from build123d import *

# Parameters (mm, degrees)
F1_DEPTH      = 76.2
F2_W          = 50.8
F2_H          = 25.4
F3_DEPTH      = 50.801
F3_DEPTH_BACK = 50.801
F5_DEPTH      = 25.4
F6_DEPTH      = 25.4
F7_W          = 25.4
F7_H          = 25.4968867362
F8_DEPTH      = 101.6
F9_R          = 12.7


with BuildPart() as f1:
    # F0 (on Top) → F1 (new body)
    with BuildSketch(Plane.XY):
        Polygon((-50.8, 101.6), (0, 0), (50.8, 101.6), align=None)
    extrude(amount=F1_DEPTH)

    # F2 (on Right) → F3 (cut, two sides)
    with BuildSketch(Plane.YZ) as f3_sk:
        with Locations((25.4, 38.1)):
            Rectangle(F2_W, F2_H)
    extrude(amount=-F3_DEPTH, mode=Mode.SUBTRACT)
    extrude(f3_sk.sketch, amount=F3_DEPTH_BACK, mode=Mode.SUBTRACT)

    # F4 (on face) → F5 (join)
    with BuildSketch(Plane(origin=(0, 0, 0), x_dir=(1, 0, 0), z_dir=(0, 0, -1))):
        with BuildLine():
            Line((63.5, -31.75), (101.6, -31.75))
            Line((101.6, -31.75), (101.6, -12.7))
            ThreePointArc((101.6, -12.7), (97.8802561211, -3.7197438789), (88.9, 0))
            Line((88.9, 0), (-88.9, 0))
            ThreePointArc((-88.9, 0), (-97.8802561211, -3.7197438789), (-101.6, -12.7))
            Line((-101.6, -12.7), (-101.6, -31.75))
            Line((-101.6, -31.75), (-63.5, -31.75))
            Line((-63.5, -31.75), (-63.5, -69.85))
            Line((-63.5, -69.85), (-101.6, -69.85))
            Line((-101.6, -69.85), (-101.6, -88.9))
            ThreePointArc((-101.6, -88.9), (-97.8802561211, -97.8802561211), (-88.9, -101.6))
            Line((-88.9, -101.6), (-50.8, -101.6))
            Line((-50.8, -101.6), (50.8, -101.6))
            Line((50.8, -101.6), (88.9, -101.6))
            ThreePointArc((88.9, -101.6), (97.8802561211, -97.8802561211), (101.6, -88.9))
            Line((101.6, -88.9), (101.6, -69.85))
            Line((101.6, -69.85), (63.5, -69.85))
            Line((63.5, -69.85), (63.5, -31.75))
        make_face()
    extrude(amount=F5_DEPTH)

    # F4 (on face) → F6 (join)
    with BuildSketch(Plane(origin=(0, 0, 0), x_dir=(1, 0, 0), z_dir=(0, 0, -1))):
        with BuildLine():
            Line((63.5, -31.75), (101.6, -31.75))
            Line((101.6, -31.75), (101.6, -12.7))
            ThreePointArc((101.6, -12.7), (97.8802561211, -3.7197438789), (88.9, 0))
            Line((88.9, 0), (-88.9, 0))
            ThreePointArc((-88.9, 0), (-97.8802561211, -3.7197438789), (-101.6, -12.7))
            Line((-101.6, -12.7), (-101.6, -31.75))
            Line((-101.6, -31.75), (-63.5, -31.75))
            Line((-63.5, -31.75), (-63.5, -69.85))
            Line((-63.5, -69.85), (-101.6, -69.85))
            Line((-101.6, -69.85), (-101.6, -88.9))
            ThreePointArc((-101.6, -88.9), (-97.8802561211, -97.8802561211), (-88.9, -101.6))
            Line((-88.9, -101.6), (-50.8, -101.6))
            Line((-50.8, -101.6), (50.8, -101.6))
            Line((50.8, -101.6), (88.9, -101.6))
            ThreePointArc((88.9, -101.6), (97.8802561211, -97.8802561211), (101.6, -88.9))
            Line((101.6, -88.9), (101.6, -69.85))
            Line((101.6, -69.85), (63.5, -69.85))
            Line((63.5, -69.85), (63.5, -31.75))
        make_face()
    extrude(amount=F6_DEPTH)

    # F7 (on face) → F8 (join)
    with BuildSketch(Plane.XZ):
        with Locations((-50.8, -38.1484433681)):
            Rectangle(F7_W, F7_H)
        with Locations((50.8, -38.1484433681)):
            Rectangle(F7_W, F7_H)
    extrude(amount=-F8_DEPTH)

    # F9
    f9_edges = [f1.edges().sort_by_distance(p)[0] for p in [
        (-38.1, 50.8, -25.4),
        (38.1, 50.8, -25.4),
    ]]
    fillet(f9_edges, radius=F9_R)


solid = f1.part
Source: CAD feature listing. Evaluate the final solid. Frame: model axes, mm. A direction names the side the tool comes from. Round coordinates to 2 decimals unless told otherwise and drop trailing zeros. Loops run counter-clockwise (first coordinate to the right, second up) from the corner with the lowest first, then second, coordinate; pieces in that order, holes last. Notation, with made-up numbers: (20, 46) - (34, 46) arc R25 cw to (34, 82) - close; hole circle Ø3 at (-22.5, 11.5). An arc over 180 degrees is marked (long way). Write item = value, one per line. Start each with the question number.
Item 1: Section query B-B on y = 47.5. Output: boundary loops of the cut face in (x, z), plus the area to 3 significant figures.
Item 2: Material intervals for line 1 (Z direction, x = -10.5, y = 25); line 2 (X direction, y = 45.5, z = -44); line 3 (Z direction, x = 7, y = 71), sorted ascending.
Item 3: Reachability of faces 4 (the face through (-26, 52, 38)), 5 (the face through (-83, 31.75, -13)), 6 (the face through (-83, 16, -25.4)), 7 (the face through (0, 31, 25.4)) from +Z, -Z, +X, -X, +Y, -Y: full face, straight path, thin tool, end or side. Return the list, or none.
Item 4: Section query C-C on y = 58.5. Output: boundary loops of the cut face in (x, z), plus the area to 3 significant figures.
Item 5: Section query A-A on x = 68. Output: boundary loops of the cut face in (y, z), plus the area to 3 significant figures.
Item 6: First-contact query: pin 1 Ø15 at (x, y) = (4, 59.5) entering from -Z; pin 2 Ø4 at (y, z) = (71, -46) entering from +X; pin 3 Ø10 at (y, z) = (42, 49.5) entering from +X. Flat tips, straight axial feed; report the tip coordinate or a pass-through.
Item 7: Mould query, pull axis X, two halves, no side actions, for faces 1 (the face through (82, 86, -25.4)), 2 (the face through (34.28, 51.51, -29.02)), 3 (the face through (101.6, 22, -13)). Classes: released by +X, released by -X, zero draft, split by the parting line, or undercut.
Item 8: Section query D-D on z = -21.5. Output: boundary loops of the cut face in (x, y), plus the area to 3 significant figures.
Results list:
q1.outline = (-63.5, -50.9) - (-38.1, -50.9) - (-38.1, -38.1) arc R12.7 cw to (-25.4, -25.4) - (25.4, -25.4) arc R12.7 cw to (38.1, -38.1) - (38.1, -50.9) - (63.5, -50.9) - (63.5, 0) - (23.75, 0) - (23.75, 25.4) - (-23.75, 25.4) - (-23.75, 0) - (-63.5, 0) - close; (-23.75, 50.8) - (23.75, 50.8) - (23.75, 76.2) - (-23.75, 76.2) - close
q1.area = 7,000 mm²
q2.line_1 = -25.4 to 25.4, 50.8 to 76.2
q2.line_2 = -63.5 to -38.1, 38.1 to 63.5
q2.line_3 = -25.4 to 76.2
q3.face_4 = +Z, -X, -Y
q3.face_5 = +Z, -Z, -X
q3.face_6 = -Z, -X, +Y, -Y
q3.face_7 = +X, -X, -Y
q4.outline = (-63.5, -50.9) - (-38.1, -50.9) - (-38.1, -38.1) arc R12.7 cw to (-25.4, -25.4) - (25.4, -25.4) arc R12.7 cw to (38.1, -38.1) - (38.1, -50.9) - (63.5, -50.9) - (63.5, 0) - (29.25, 0) - (29.25, 76.2) - (-29.25, 76.2) - (-29.25, 0) - (-63.5, 0) - close
q4.area = 9,050 mm²
q5.outline = (0, -25.4) - (31.75, -25.4) - (31.75, 0) - (0, 0) - close; (69.85, -25.4) - (101.6, -25.4) - (101.6, 0) - (69.85, 0) - close
q5.area = 1,610 mm²
q6.pin_1 = -25.4
q6.pin_2 = 63.5
q6.pin_3 = 23.41
q7.face_1 = zero draft
q7.face_2 = undercut
q7.face_3 = released by +X
q8.outline = (-101.6, 12.7) arc R12.7 ccw to (-88.9, 0) - (88.9, 0) arc R12.7 ccw to (101.6, 12.7) - (101.6, 31.75) - (63.5, 31.75) - (63.5, 69.85) - (101.6, 69.85) - (101.6, 88.9) arc R12.7 ccw to (88.9, 101.6) - (-88.9, 101.6) arc R12.7 ccw to (-101.6, 88.9) - (-101.6, 69.85) - (-63.5, 69.85) - (-63.5, 31.75) - (-101.6, 31.75) - close
q8.area = 17,600 mm²
